Check sheet for the modelled part. Datum: model origin and axes. Units: mm. A direction names the side the tool comes from. Give positions to 0.01 mm unless a question says otherwise; leave off trailing zeros. Order: outer loops, then holes, each group sorted by start corner. A loop starts at its lowest first (then second) coordinate and runs counter-clockwise, first axis right, second up. Notation, with made-up numbers: (27.25, 78) -> (53.25, 78) arc R15 cw to (53.25, 86) -> close; hole circle Ø4 at (1, -7). An arc over 180 degrees is marked (long way). One line per question, with ' | ' between items.
```python
from build123d import *

# Parameters (mm, degrees)
F1_DEPTH = 3
F4_DEPTH = 4
F5_W     = 3
F5_H     = 25
F6_DEPTH = 15
F8_R     = 1.5
F9_DEPTH = 6


with BuildPart() as f1:
    # F0 (on Front) → F1 (new body)
    with BuildSketch(Plane.XZ):
        with BuildLine():
            Line((-17.0412734266, 17.0412734266), (-21, 21))
            Line((-21, 21), (-21, -21))
            Line((-21, -21), (-17.0412734266, -17.0412734266))
            ThreePointArc((-17.0412734266, -17.0412734266), (-17.0412734266, -14.7785317268), (-14.7785317268, -14.7785317268))
            Line((-14.7785317268, -14.7785317268), (-8.1317279836, -8.1317279836))
            ThreePointArc((-8.1317279836, -8.1317279836), (-11.5, 0), (-8.1317279836, 8.1317279836))
            Line((-8.1317279836, 8.1317279836), (-14.7785317268, 14.7785317268))
            ThreePointArc((-14.7785317268, 14.7785317268), (-17.0412734266, 14.7785317268), (-17.0412734266, 17.0412734266))
        make_face()
        with BuildLine():
            Line((21, 21), (-21, 21))
            Line((-21, 21), (-17.0412734266, 17.0412734266))
            ThreePointArc((-17.0412734266, 17.0412734266), (-15.2976090849, 17.3881098287), (-14.3099025767, 15.9099025767))
            ThreePointArc((-14.3099025767, 15.9099025767), (-14.4316953247, 15.2976090849), (-14.7785317268, 14.7785317268))
            Line((-14.7785317268, 14.7785317268), (-8.1317279836, 8.1317279836))
            ThreePointArc((-8.1317279836, 8.1317279836), (0, 11.5), (8.1317279836, 8.1317279836))
            Line((8.1317279836, 8.1317279836), (14.7785317268, 14.7785317268))
            ThreePointArc((14.7785317268, 14.7785317268), (14.7785317268, 17.0412734266), (17.0412734266, 17.0412734266))
            Line((17.0412734266, 17.0412734266), (21, 21))
        make_face()
        with BuildLine():
            Line((21, -21), (21, 21))
            Line((21, 21), (17.0412734266, 17.0412734266))
            ThreePointArc((17.0412734266, 17.0412734266), (17.3881098287, 16.5221960685), (17.5099025767, 15.9099025767))
            ThreePointArc((17.5099025767, 15.9099025767), (16.5221960685, 14.4316953247), (14.7785317268, 14.7785317268))
            Line((14.7785317268, 14.7785317268), (8.1317279836, 8.1317279836))
            ThreePointArc((8.1317279836, 8.1317279836), (10.6246146239, 4.4008594722), (11.5, 0))
            ThreePointArc((11.5, 0), (10.6246146239, -4.4008594722), (8.1317279836, -8.1317279836))
            Line((8.1317279836, -8.1317279836), (14.7785317268, -14.7785317268))
            ThreePointArc((14.7785317268, -14.7785317268), (16.5221960685, -14.4316953247), (17.5099025767, -15.9099025767))
            ThreePointArc((17.5099025767, -15.9099025767), (17.3881098287, -16.5221960685), (17.0412734266, -17.0412734266))
            Line((17.0412734266, -17.0412734266), (21, -21))
        make_face()
        with BuildLine():
            Line((-17.0412734266, -17.0412734266), (-21, -21))
            Line((-21, -21), (21, -21))
            Line((21, -21), (17.0412734266, -17.0412734266))
            ThreePointArc((17.0412734266, -17.0412734266), (14.7785317268, -17.0412734266), (14.7785317268, -14.7785317268))
            Line((14.7785317268, -14.7785317268), (8.1317279836, -8.1317279836))
            ThreePointArc((8.1317279836, -8.1317279836), (0, -11.5), (-8.1317279836, -8.1317279836))
            Line((-8.1317279836, -8.1317279836), (-14.7785317268, -14.7785317268))
            ThreePointArc((-14.7785317268, -14.7785317268), (-14.4316953247, -15.2976090849), (-14.3099025767, -15.9099025767))
            ThreePointArc((-14.3099025767, -15.9099025767), (-15.2976090849, -17.3881098287), (-17.0412734266, -17.0412734266))
        make_face()
    extrude(amount=F1_DEPTH)

    # F3 (on offset) → F4 (join)
    with BuildSketch(Plane.XY.offset(21)):
        Polygon((0, 0), (-21, 0), (-21, -15), (-12.5, -15), (-12.5, -30), (0, -30), align=None)
        Polygon((21, 0), (0, 0), (0, -30), (12.5, -30), (12.5, -15), (21, -15), align=None)
    extrude(amount=F4_DEPTH)

    # F5 (on Front) → F6 (join)
    with BuildSketch(Plane.XZ):
        with Locations((-22.5, 12.5)):
            Rectangle(F5_W, F5_H)
        with Locations((22.5, 12.5)):
            Rectangle(F5_W, F5_H)
    extrude(amount=F6_DEPTH)

    # F8 (on offset) → F9 (join)
    with BuildSketch(Plane(origin=(0, 0, 0), x_dir=(1, 0, 0), z_dir=(0, 0, -1))):
        with BuildLine():
            Line((24, 0), (31.2, 9.6))
            ThreePointArc((31.2, 9.6), (31.2887687666, 14.2768399153), (26.88, 15.84))
            Line((26.88, 15.84), (24, 15))
            Line((24, 15), (24, 0))
        make_face()
        with Locations((28, 12)):
            Circle(F8_R, mode=Mode.SUBTRACT)
        with BuildLine():
            Line((-24, 0), (-24, 15))
            Line((-24, 15), (-26.88, 15.84))
            ThreePointArc((-26.88, 15.84), (-31.2887687666, 14.2768399153), (-31.2, 9.6))
            Line((-31.2, 9.6), (-24, 0))
        make_face()
        with Locations((-28, 12)):
            Circle(F8_R, mode=Mode.SUBTRACT)
    extrude(amount=-F9_DEPTH)


solid = f1.part
```
Q1. Depth check by flat-ended pin: pin 1 Ø13 at (y, z) = (-6, 11) entering from +X; pin 2 Ø4.5 at (y, z) = (-6, 17) entering from -X; pin 3 Ø1 at (x, z) = (25, 1.5) entering from -Y. Enter the tip coordinate at first touch or a pass-through.
Result sheet:
pin 1: stops at x = 31.55 | pin 2: stops at x = -24 | pin 3: stops at y = -15.44
Q2. Mould release check, pull along X, two halves, no side actions. Record for faces 6 (the face through (0, -13, 21)), 7 (the face through (-24, -7, 15)), 8 (the face through (27.55, -4.73, 2.96)): pulls with the +X half, pulls with the -X half, needs draft (parallel to the pull), parting line crosses it, or undercut.
Result sheet:
face 6: undercut | face 7: pulls with the -X half | face 8: pulls with the +X half
Q3. Access from +Z, -Z, +X, -X, +Y, -Y to the whole of each face (thin tool, end or side, straight path). Record for faces 1 (the face through (21.2, -15, 15.2)), 2 (the face through (-10, -3, 10)), 3 (the face through (27, -10, 6)), 4 (the face through (-12.5, -22, 23)), 5 (the face through (25, -10, 0)).
Result sheet:
face 1: +Z, -Z, -Y | face 2: -Z, -Y | face 3: +Z, +X, +Y, -Y | face 4: +Z, -Z, -X, -Y | face 5: -Z, +X, +Y, -Y
Q4. Section check D-D (x = 13.5). Enter the section's corners in (y, z), and give its area (3 significant figures).
Result sheet:
outline: (-15, 21) -> (-3, 21) -> (-3, -21) -> (0, -21) -> (0, 25) -> (-15, 25) -> close | area: 186 mm2
Q5. Section check A-A (y = -12). Enter the section's corners in (x, z).
Result sheet:
outline: (-32, 0) -> (-29.5, 0) -> (-29.5, 6) -> (-32, 6) -> close; (-26.5, 0) -> (-21, 0) -> (-21, 21) -> (21, 21) -> (21, 0) -> (26.5, 0) -> (26.5, 6) -> (24, 6) -> (24, 25) -> (-24, 25) -> (-24, 6) -> (-26.5, 6) -> close; (29.5, 0) -> (32, 0) -> (32, 6) -> (29.5, 6) -> close
Q6. Section check C-C (x = 2.5). Enter the section's corners in (y, z).
Result sheet:
outline: (-30, 21) -> (-3, 21) -> (-3, 11.22) -> (0, 11.22) -> (0, 25) -> (-30, 25) -> close; (-3, -21) -> (0, -21) -> (0, -11.22) -> (-3, -11.22) -> close
Q7. Section check B-B (z = 2). Enter the section's corners in (x, y).
Result sheet:
outline: (-31.2, -9.6) arc R4 ccw to (-26.88, -15.84) -> (-24, -15) -> (-21, -15) -> (-21, -3) -> (-11.32, -3) -> (-11.32, 0) -> (-24, 0) -> close; (11.32, -3) -> (21, -3) -> (21, -15) -> (24, -15) -> (26.88, -15.84) arc R4 ccw to (31.2, -9.6) -> (24, 0) -> (11.32, 0) -> close; hole circle Ø3 at (-28, -12); hole circle Ø3 at (28, -12)
Q8. Thickness scan on line 1 (X direction, y = -12, z = 2.2); line 2 (X direction, y = -12, z = 7); line 3 (Y direction, x = -28, z = 4). Record the ranges inside material, lowest first.
Result sheet:
line 1: x = -32 to -29.5, -26.5 to -21, 21 to 26.5, 29.5 to 32 | line 2: x = -24 to -21, 21 to 24 | line 3: y = -16 to -13.5, -10.5 to -5.33
